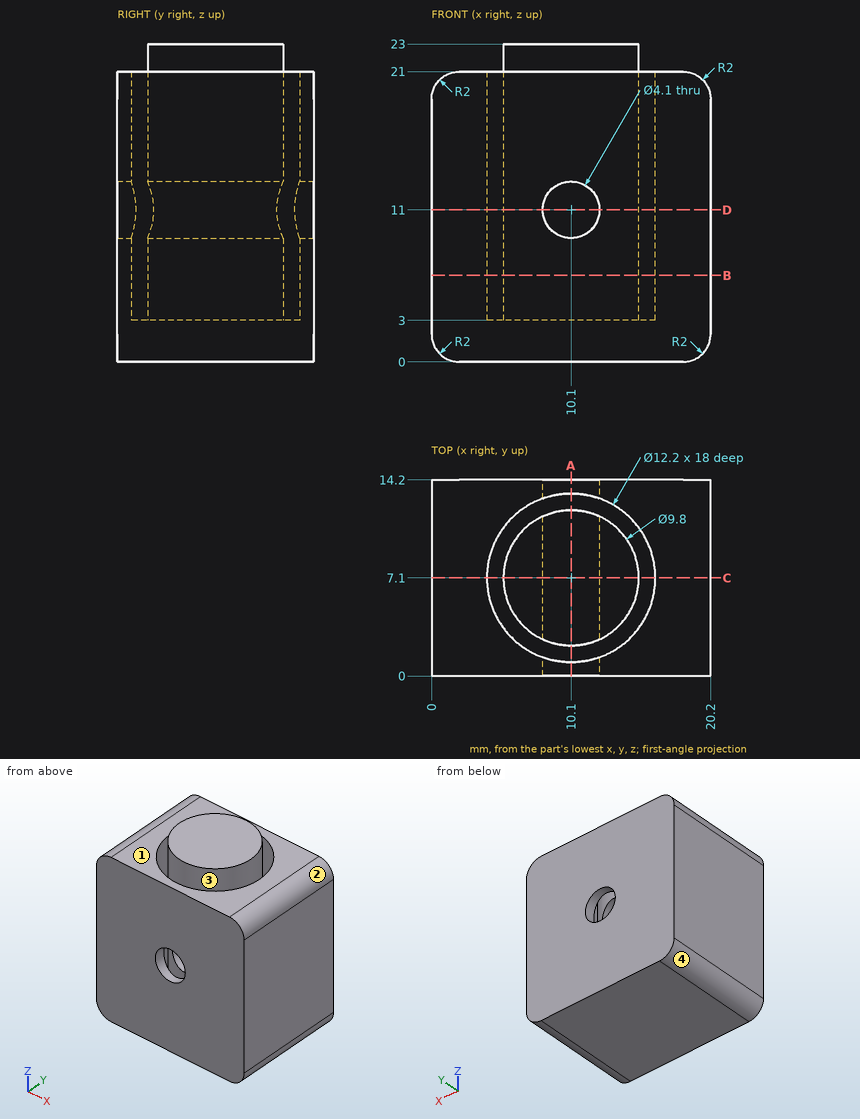
Check sheet for the drawn part. Datum: minimum x, y, z corner. Units: mm. Round coordinates to 2 decimals unless told otherwise and drop trailing zeros. Order: outer loops, then holes, each group sorted by start corner. A loop starts at its lowest first (then second) coordinate and runs counter-clockwise, first axis right, second up.
1) Mould release check, pull along X, two halves, no side actions. Record for the marked faces 1, 2, 3 and 4: +X half, -X half, draft (parallel to the pull), parting line (faces both ways), or undercut.
2) Section check B-B (z = 6.25). Record the boundary of the cut face in (x, y).
3) Scan lines: line 1 (X direction, y = 11.5, z = 5); line 2 (Y direction, x = 10.5, z = 18.75); line 3 (Z direction, x = 10.1, y = 13.6). Record each from-to range of solid material in increasing order.
4) Section check A-A (x = 10.1). Record the boundary of the cut face in (y, z), and give its area (3 significant figures).
5) Section check D-D (z = 11). Record the boundary of the cut face in (x, y), and give its area (3 significant figures).
6) Section check C-C (y = 7.1). Record the boundary of the cut face in (x, z).
Result:
1. face 1: draft
1. face 2: +X half
1. face 3: undercut
1. face 4: -X half
2. outline: (0, 0) - (20.2, 0) - (20.2, 14.2) - (0, 14.2) - close; circle Ø9.8 at (10.1, 7.1); hole circle Ø12.2 at (10.1, 7.1)
3. line 1: x = 0 to 5.88, 7.94 to 12.26, 14.32 to 20.2
3. line 2: y = 0 to 1.01, 2.22 to 11.98, 13.19 to 14.2
3. line 3: z = 0 to 8.95, 13.05 to 21
4. outline: (0, 0) - (14.2, 0) - (14.2, 8.95) - (13.2, 8.95) - (13.2, 3) - (12, 3) - (12, 8.95) - (2.2, 8.95) - (2.2, 3) - (1, 3) - (1, 8.95) - (0, 8.95) - close; (0, 13.05) - (1, 13.05) - (1, 21) - (0, 21) - close; (2.2, 13.05) - (12, 13.05) - (12, 23) - (2.2, 23) - close; (13.2, 13.05) - (14.2, 13.05) - (14.2, 21) - (13.2, 21) - close
4. area: 226 mm2
5. outline: (0, 0) - (8.05, 0) - (8.05, 1.35) arc R6.1 cw to (8.05, 12.85) - (8.05, 14.2) - (0, 14.2) - close; (8.05, 2.65) - (8.05, 11.55) arc R4.9 ccw to start; (12.15, 0) - (20.2, 0) - (20.2, 14.2) - (12.15, 14.2) - (12.15, 12.85) arc R6.1 cw to (12.15, 1.35) - close; (12.15, 2.65) arc R4.9 ccw to (12.15, 11.55) - close
5. area: 197 mm2
6. outline: (0, 2) arc R2 ccw to (2, 0) - (18.2, 0) arc R2 ccw to (20.2, 2) - (20.2, 19) arc R2 ccw to (18.2, 21) - (16.2, 21) - (16.2, 3) - (15, 3) - (15, 23) - (5.2, 23) - (5.2, 3) - (4, 3) - (4, 21) - (2, 21) arc R2 ccw to (0, 19) - close; hole circle Ø4.1 at (10.1, 11)
